Geometry: see drawing. Coordinates: mm, zero at the bounding-box minimum. Coordinates: 2 decimals unless noted, no trailing zeros. Order: outer loops, then holes, each group sorted by start corner. A loop starts at its lowest first (then second) coordinate and runs counter-clockwise, first axis right, second up.
Item 1: Section A-A on x = 25.4. Return the cut outline in (y, z).
Item 2: Contact query for flat-ended pins moving along their axis: P1, Ø3.5, axis at x = 7, y = 35, coming from the +Z side; P2, Ø3, axis at x = 190.5, z = 9, coming from the -Y side. Output: stop coordinate, or through.
Item 3: Ray query, line 1 (X direction, y = 63.5, z = 16); line 2 (Z direction, x = 190.5, y = 5); line 3 (X direction, y = 19, z = 7). Return the intervals inside material, ascending.
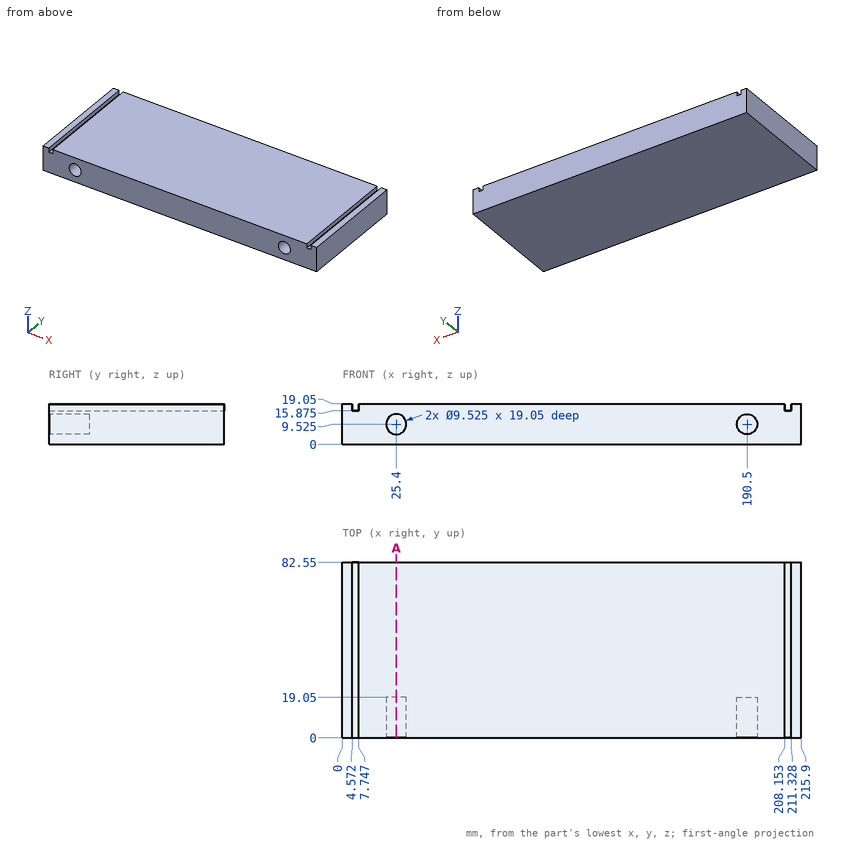
Answer list:
1. outline: (0, 0) - (82.55, 0) - (82.55, 19.05) - (0, 19.05) - (0, 14.29) - (19.05, 14.29) - (19.05, 4.76) - (0, 4.76) - close
2. P1: stops at z = 19.05
2. P2: stops at y = 19.05
3. line 1: x = 0 to 4.57, 7.75 to 208.15, 211.33 to 215.9
3. line 2: z = 0 to 4.76, 14.29 to 19.05
3. line 3: x = 0 to 21.36, 29.44 to 186.46, 194.54 to 215.9
